from build123d import *

# Parameters (mm, degrees)
SKETCH1_R           = 10
BOSS_EXTRUDE1_DEPTH = 15
SKETCH3_R           = 8.5
CUT_EXTRUDE1_DEPTH  = 19
SKETCH4_W           = 1
SKETCH4_H           = 15
CUT_EXTRUDE3_DEPTH  = 3


with BuildPart() as part:
    # Sketch1 → Boss-Extrude1 (new body)
    with BuildSketch(Plane.XY):
        Circle(SKETCH1_R)
    extrude(amount=BOSS_EXTRUDE1_DEPTH)

    # Sketch3 → Cut-Extrude1 (cut)
    with BuildSketch(Plane.XY.offset(15)):
        Circle(SKETCH3_R)
    extrude(amount=-CUT_EXTRUDE1_DEPTH, mode=Mode.SUBTRACT)

    # Sketch4 → Cut-Extrude3 (cut)
    with BuildSketch(Plane(origin=(0, 8, 0), x_dir=(1, 0, 0), z_dir=(0, 1, 0))):
        with Locations((-0.265251336, -7.5)):
            Rectangle(SKETCH4_W, SKETCH4_H)
    extrude(amount=CUT_EXTRUDE3_DEPTH, mode=Mode.SUBTRACT)


solid = part.part
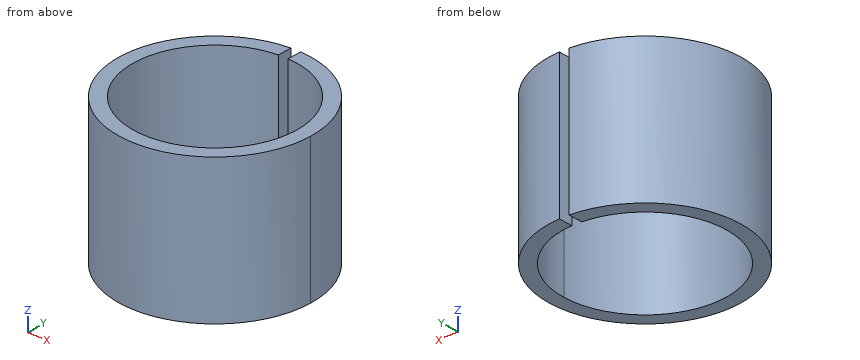
The listing builds one solid part. Answer for the finished solid, in the listing's coordinates (mm). Give positions to 0.01 mm unless a question says otherwise; leave off trailing zeros. Write each loop counter-clockwise with the first axis right and the second up, starting at its lowest first coordinate (ties: lowest second). Pieces come first, ordered by that corner, then holes. Notation, with made-up numbers: (79.5, 51) -> (88.5, 51) arc R17 cw to (88.5, 60) -> close; hole circle Ø1 at (2.25, 34.25). An arc over 180 degrees is marked (long way). One line per question, with ' | ' between items. Start each with the question number.
1. Section C-C (z = 4) is taken. Determine the outline of the cut face in (x, y).
2. Section A-A (y = 0.5) is taken. Determine the outline of the cut face in (x, z).
3. Section D-D (x = -0.25) is taken. Determine the outline of the cut face in (y, z).
4. Given pin 1 Ø4 at (x, y) = (2.5, 7.5) entering from +Z; pin 2 Ø1 at (y, z) = (-3, 7.5) entering from -X; pin 3 Ø4 at (x, y) = (4.5, -1) entering from -Z; pin 4 Ø0.8 at (y, z) = (9.5, 10.5) entering from -X, each flat-ended and moving along its own axis, determine where each tip first touches the part or whether it passes through.
5. Section B-B (x = 7.5) is taken. Determine the outline of the cut face in (y, z), plus the area to 3 significant figures.
6. Find the intervals of material crossed by probe 1 along X at (y, z) = (0, 6); probe 2 along Y at (x, z) = (0, 3.5); probe 3 along X at (y, z) = (4, 11), in increasing order.
Response values:
1) outline: (-0.77, 8.47) -> (-0.77, 9.97) arc R10 ccw (long way) to (0.23, 10) -> (0.23, 8.5) arc R8.5 cw (long way) to start
2) outline: (-9.99, 0) -> (-8.49, 0) -> (-8.49, 15) -> (-9.99, 15) -> close; (8.49, 0) -> (9.99, 0) -> (9.99, 15) -> (8.49, 15) -> close
3) outline: (-10, 0) -> (-8.5, 0) -> (-8.5, 15) -> (-10, 15) -> close
4) pin 1: z = 15 | pin 2: x = -9.68 | pin 3: through | pin 4: x = -4.15
5) outline: (-6.61, 0) -> (-4, 0) -> (-4, 15) -> (-6.61, 15) -> close; (4, 0) -> (6.61, 0) -> (6.61, 15) -> (4, 15) -> close | area: 78.4 mm2
6) probe 1: -10 to -8.5, 8.5 to 10 | probe 2: -10 to -8.5 | probe 3: -9.17 to -7.5, 7.5 to 9.17
